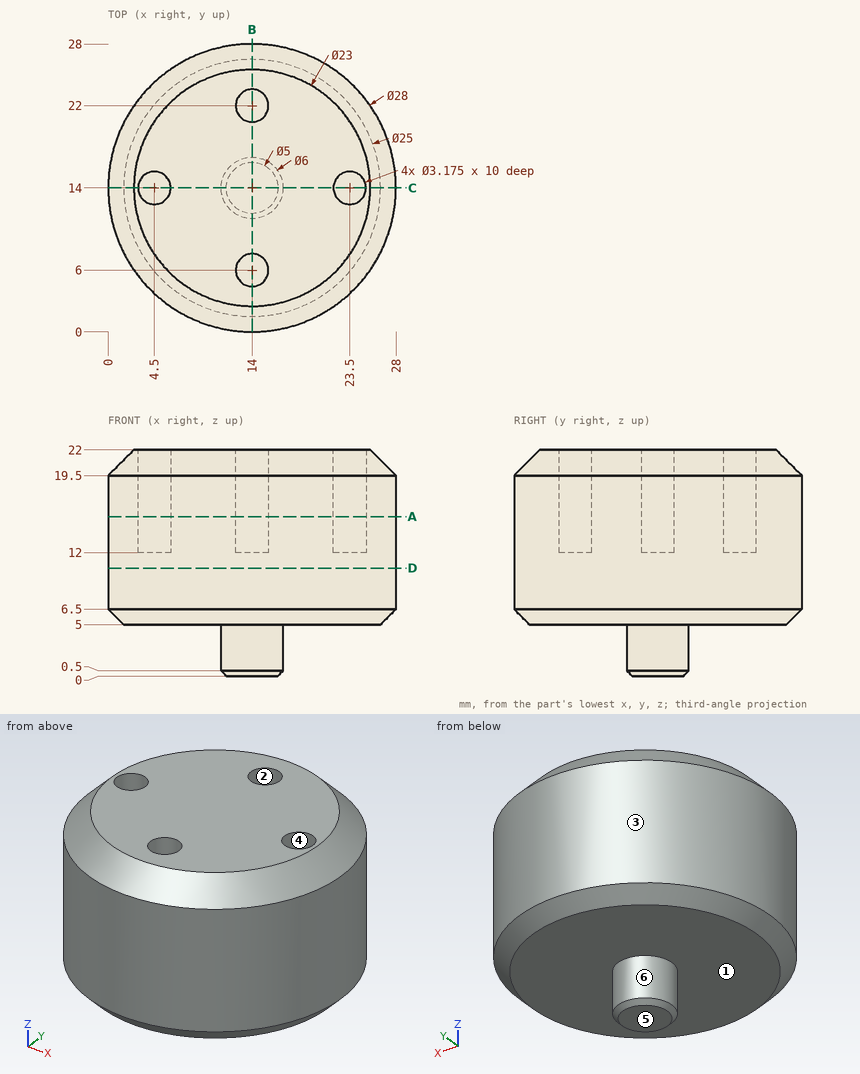
Could you check a few things on this drawing? It's one solid part, dimensions in mm from its lowest x, y, z. A direction names the side the tool comes from. Give positions to 0.01 mm unless a question says otherwise; leave off trailing zeros. Order: outer loops, then holes, each group sorted by start corner. A loop starts at its lowest first (then second) coordinate and runs counter-clockwise, first axis right, second up. Notation, with made-up numbers: (44, 84) - (63, 84) arc R22 ccw to (63, 98) - close; hole circle Ø8 at (16, -3.5). An arc over 180 degrees is marked (long way). Return JSON: item names as keys, results as strings. Group by question number.
Q1. Thinking about a two-plate mould opening in Y: for the marked faces 1, 2 and 3, which applies, pulls with the +Y half, pulls with the -Y half, needs draft (parallel to the pull), parting line crosses it, or undercut?
Q2. Will these pins go through, and if not, where does the flat tip stop? pin 1 Ø3 at (x, z) = (4, 7.5) entering from +Y; pin 2 Ø1.9 at (x, y) = (14, 6) entering from -Z; pin 3 Ø1.9 at (x, y) = (23.5, 14) entering from +Z.
Q3. Suppose I cut it at B-B, the plane x = 14. Please give me the cut outline in (y, z).
Q4. Suppose I cut it at C-C, the plane y = 14. Please give me the cut outline in (x, z).
Q5. Please list where these lines run through material, in increasing order: line 1 along Y through (x, z) = (15, 16.5); line 2 along Y through (x, z) = (13.25, 20.25); line 3 along Y through (x, z) = (4.5, 18). Write a range as [from, to].
Q6. Which directions (+Z, -Z, +X, -X, +Y, -Y) give clear straight access to the entire face, cutting with the end or side of a thin tool? Please do the marked faces 4, 5 and 6.
Q7. Suppose I cut it at D-D, the plane z = 10.5. Please give me the cut outline in (x, y).
Q8. Suppose I cut it at A-A, the plane z = 15.5. Please give me the cut outline in (x, y) (1 decimal).
Resolved:
{
 "1": {"face 1": "needs draft", "face 2": "undercut", "face 3": "parting line crosses it"},
 "2": {"pin 1": "stops at y = 25.12", "pin 2": "stops at z = 5", "pin 3": "stops at z = 12"},
 "3": {"outline": "(0, 6.5) - (1.5, 5) - (11, 5) - (11, 0.5) - (11.5, 0) - (16.5, 0) - (17, 0.5) - (17, 5) - (26.5, 5) - (28, 6.5) - (28, 19.5) - (25.5, 22) - (23.59, 22) - (23.59, 12) - (20.41, 12) - (20.41, 22) - (7.59, 22) - (7.59, 12) - (4.41, 12) - (4.41, 22) - (2.5, 22) - (0, 19.5) - close"},
 "4": {"outline": "(0, 6.5) - (1.5, 5) - (11, 5) - (11, 0.5) - (11.5, 0) - (16.5, 0) - (17, 0.5) - (17, 5) - (26.5, 5) - (28, 6.5) - (28, 19.5) - (25.5, 22) - (25.09, 22) - (25.09, 12) - (21.91, 12) - (21.91, 22) - (6.09, 22) - (6.09, 12) - (2.91, 12) - (2.91, 22) - (2.5, 22) - (0, 19.5) - close"},
 "5": {"line 1": "y = [0.04, 4.77], [7.23, 20.77], [23.23, 27.96]", "line 2": "y = [0.77, 4.6], [7.4, 20.6], [23.4, 27.23]", "line 3": "y = [3.72, 12.41], [15.59, 24.28]"},
 "6": {"face 4": "+Z", "face 5": "-Z, +X, -X, +Y, -Y", "face 6": "-Z"},
 "7": {"outline": "circle Ø28 at (14, 14)"},
 "8": {"outline": "circle Ø28 at (14, 14); hole circle Ø3.2 at (4.5, 14); hole circle Ø3.2 at (14, 6); hole circle Ø3.2 at (14, 22); hole circle Ø3.2 at (23.5, 14)"}
}
